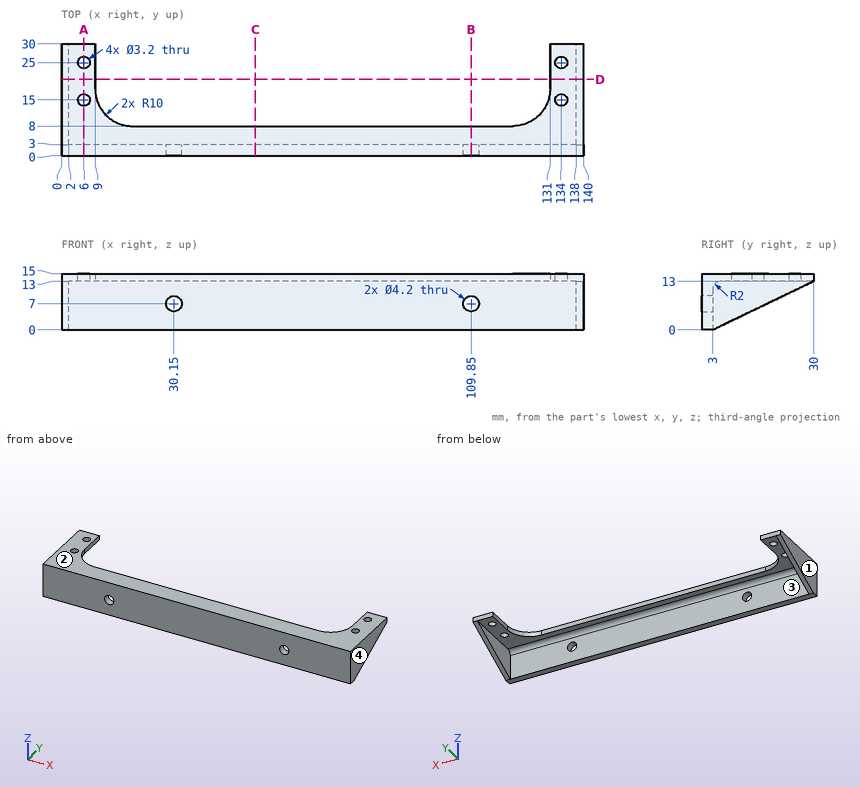
Could you check a few things on this drawing? It's one solid part, dimensions in mm from its lowest x, y, z. Round coordinates to 2 decimals unless told otherwise and drop trailing zeros. Loops run counter-clockwise (first coordinate to the right, second up) from the corner with the lowest first, then second, coordinate; pieces in that order, holes last. Notation, with made-up numbers: (33.5, 60) -> (47.5, 60) arc R24 cw to (47.5, 98) -> close; hole circle Ø5 at (42.5, 63.25). An arc over 180 degrees is marked (long way). One line per item, written item: value. Start each with the question number.
1. If we section it at B-B, the plane x = 109.85: Write out the boundary of the cut face in (y, z), then the cut area to 3 significant figures.
2. If we section it at C-C, the plane x = 52: Write out the boundary of the cut face in (y, z).
3. If we section it at A-A, the plane x = 6: Write out the boundary of the cut face in (y, z), then the cut area to 3 significant figures.
4. If we section it at D-D, the plane y = 20.5: Write out the boundary of the cut face in (x, z), then the cut area to 3 significant figures.
5. For pin 1 (3.5 mm diameter, centred on x = 48, z = 7.5, fed in from +Y); pin 2 (3.5 mm diameter, centred on x = 6, y = 25, fed in from -Z); pin 3 (1 mm diameter, centred on x = 53, z = 13.5, fed in from +Y), each with a flat end and sliding along its axis, tell me the tip position at first contact or that it passes through.
6. If I drill on probe 1 along X at (y, z) = (1.5, 7); probe 2 along Y at (x, z) = (134, 14.2); probe 3 along X at (y, z) = (9, 12.25), over which ranges is the centre line in solid material (lowest first)?
7. If we mould it in two halves opening along X, with no side actions, what happens to the marked faces 1, 2, 3 and 4? For each: pulls with the +X half, pulls with the -X half, needs draft (parallel to the pull), parting line crosses it, or undercut.
Calculated:
1. outline: (0, 0) -> (3, 0) -> (3, 4.9) -> (0, 4.9) -> close; (0, 9.1) -> (3, 9.1) -> (3, 11) arc R2 cw to (5, 13) -> (8, 13) -> (8, 15) -> (0, 15) -> close
1. area: 43.3 mm²
2. outline: (0, 0) -> (3, 0) -> (3, 11) arc R2 cw to (5, 13) -> (8, 13) -> (8, 15) -> (0, 15) -> close
3. outline: (0, 0) -> (3, 0) -> (3, 11) arc R2 cw to (5, 13) -> (13.4, 13) -> (13.4, 15) -> (0, 15) -> close; (16.6, 13) -> (23.4, 13) -> (23.4, 15) -> (16.6, 15) -> close; (26.6, 13) -> (30, 13) -> (30, 15) -> (26.6, 15) -> close
3. area: 87.1 mm²
4. outline: (0, 8.43) -> (2, 8.43) -> (2, 13) -> (9, 13) -> (9, 15) -> (0, 15) -> close; (131, 13) -> (138, 13) -> (138, 8.43) -> (140, 8.43) -> (140, 15) -> (131, 15) -> close
4. area: 54.3 mm²
5. pin 1: stops at y = 3
5. pin 2: stops at z = 13
5. pin 3: stops at y = 8
6. probe 1: x = 0 to 28.05, 32.25 to 107.75, 111.95 to 140
6. probe 2: y = 0 to 13.4, 16.6 to 23.4, 26.6 to 30
6. probe 3: x = 0 to 2, 138 to 140
7. face 1: pulls with the -X half
7. face 2: needs draft
7. face 3: undercut
7. face 4: pulls with the +X half
